Verification items for the finished model (mm, model axes). A direction names the side the tool comes from. Give positions to 0.01 mm unless a question says otherwise; leave off trailing zeros. Loops run counter-clockwise (first coordinate to the right, second up) from the corner with the lowest first, then second, coordinate; pieces in that order, holes last. Notation, with made-up numbers: (16, 74) - (68, 74) arc R16 ccw to (68, 80) - close; hole circle Ø3 at (75, 54). An arc over 180 degrees is marked (long way). One line per question, with ' | ' between items. Start each with the question number.
1. Section check B-B, the plane z = 560.5. Enter the section's corners in (x, y), then the cut area to 3 significant figures.
2. Tool access check on faces 5 (the face through (-31.75, 0, 701)), 6 (the face through (0, -29.642, 701)). Record the directions out of +Z, -Z, +X, -X, +Y, -Y that give a thin tool (end or side, any length) a straight path to the whole face; none if there is none.
3. Mould release check, pull along Y, two halves, no side actions. Record for faces 1 (the face through (0, 31.75, 701)), 2 (the face through (0, -31.75, 701)), 3 (the face through (0, -30, 1422.4)), 4 (the face through (29.642, 0, 701)): +Y half, -Y half, draft (parallel to the pull), parting line (faces both ways), or undercut.
4. Thickness scan on line 1 along Y through (x, z) = (9.5, 439.5). Record the ranges inside material, lowest first. Write a range as from..to.
5. Depth check by flat-ended pin: pin 1 Ø8 at (y, z) = (9.525, 92.075) entering from +X. Enter the tip coordinate at first touch or a pass-through.
6. Section check A-A, the plane y = -12. Enter the section's corners in (x, z).
from build123d import *

# Parameters (mm, degrees)
BOSS_EXTRUDE1_DEPTH     = 1422.4
F_1_2_CLEARANCE_HOLE1_D = 13.09624


with BuildPart() as part:
    # Sketch1 → Boss-Extrude1 (new body)
    with BuildSketch(Plane.XY):
        with BuildLine():
            Line((27.5336, 31.75), (-27.5336, 31.75))
            ThreePointArc((-27.5336, 31.75), (-30.515045032, 30.515045032), (-31.75, 27.5336))
            Line((-31.75, 27.5336), (-31.75, -27.5336))
            ThreePointArc((-31.75, -27.5336), (-30.515045032, -30.515045032), (-27.5336, -31.75))
            Line((-27.5336, -31.75), (27.5336, -31.75))
            ThreePointArc((27.5336, -31.75), (30.515045032, -30.515045032), (31.75, -27.5336))
            Line((31.75, -27.5336), (31.75, 27.5336))
            ThreePointArc((31.75, 27.5336), (30.515045032, 30.515045032), (27.5336, 31.75))
        make_face()
        with BuildLine():
            Line((27.5336, 29.6418), (-27.5336, 29.6418))
            ThreePointArc((-27.5336, 29.6418), (-29.024322516, 29.024322516), (-29.6418, 27.5336))
            Line((-29.6418, 27.5336), (-29.6418, -27.5336))
            ThreePointArc((-29.6418, -27.5336), (-29.024322516, -29.024322516), (-27.5336, -29.6418))
            Line((-27.5336, -29.6418), (27.5336, -29.6418))
            ThreePointArc((27.5336, -29.6418), (29.024322516, -29.024322516), (29.6418, -27.5336))
            Line((29.6418, -27.5336), (29.6418, 27.5336))
            ThreePointArc((29.6418, 27.5336), (29.024322516, 29.024322516), (27.5336, 29.6418))
        make_face(mode=Mode.SUBTRACT)
    extrude(amount=BOSS_EXTRUDE1_DEPTH)

    # 1/2 Clearance Hole1 (through all)
    with Locations(Plane(origin=(31.75, 9.525, 22.225), x_dir=(0, 0, 1), z_dir=(1, 0, 0))):
        with Locations((0, 0), (69.85, 0), (139.7, 0)):
            Hole(F_1_2_CLEARANCE_HOLE1_D / 2)


solid = part.part
Results list:
1) outline: (-31.75, -27.53) arc R4.22 ccw to (-27.53, -31.75) - (27.53, -31.75) arc R4.22 ccw to (31.75, -27.53) - (31.75, 27.53) arc R4.22 ccw to (27.53, 31.75) - (-27.53, 31.75) arc R4.22 ccw to (-31.75, 27.53) - close; hole (-29.64, -27.53) arc R2.11 ccw to (-27.53, -29.64) - (27.53, -29.64) arc R2.11 ccw to (29.64, -27.53) - (29.64, 27.53) arc R2.11 ccw to (27.53, 29.64) - (-27.53, 29.64) arc R2.11 ccw to (-29.64, 27.53) - close | area: 506 mm²
2) face 5: +Z, -Z, -X, +Y, -Y | face 6: +Z, -Z
3) face 1: +Y half | face 2: -Y half | face 3: draft | face 4: undercut
4) line 1: -31.75..-29.64, 29.64..31.75
5) pin 1: through
6) outline: (-31.75, 0) - (-29.64, 0) - (-29.64, 1422.4) - (-31.75, 1422.4) - close; (29.64, 0) - (31.75, 0) - (31.75, 1422.4) - (29.64, 1422.4) - close
